Here's how the part is built. I have some questions about the finished solid (model axes, mm). A direction names the side the tool comes from. Coordinates: 2 decimals unless noted, no trailing zeros. Write each loop counter-clockwise with the first axis right and the second up, starting at its lowest first coordinate (ties: lowest second). Pieces come first, ordered by that corner, then holes.
Item 1: For faces 4 (the face through (-5.937, 13, -1)), 5 (the face through (10.444, -14.766, 1.009)), which set-ups out of +Z, -Z, +X, -X, +Y, -Y let a thin tool reach every point of the face, with its end or its side?
Item 2: If I drill on line 1 (X direction, y = -8, z = -0.5); line 2 (X direction, y = 16, z = 2.8) (3 decimals); line 3 (X direction, y = -15.5, z = 0.15), over which ranges is the centre line in solid material (lowest first)?
Item 3: If we section it at D-D (z = 3.5): Please give me the cut outline in (x, y).
Item 4: I'm going to push flat-ended pins straight in: pin 1 Ø10.5 at (x, y) = (1.5, 2.5) entering from -Z; pin 2 Ø4.5 at (x, y) = (-11.5, 1.5) entering from -Z; pin 3 Ø4.5 at (x, y) = (12.94, 14.66) entering from -Z. Where does each tip first touch, or does it pass through?
Item 5: If we section it at B-B (y = 8): Please give me the cut outline in (x, z), then the cut area to 3 significant figures.
Item 6: If we section it at A-A (x = -1.5): Please give me the cut outline in (y, z).
Item 7: We'd pull the mould along Y, two halves only. Please class faces 1 (the face through (-0.79, -11.52, 1.97)), 2 (the face through (-18.713, 0, 1)), 3 (the face through (0, -19.656, 1)): +Y half, -Y half, draft (parallel to the pull), parting line (faces both ways), or undercut.
Item 8: If we section it at C-C (z = 1.5): Please give me the cut outline in (x, y), then the cut area to 3 significant figures.
from build123d import *

# Parameters (mm, degrees)
SKETCH1_W           = 36.654989836
SKETCH1_H           = 39.3126
SKETCH1_R           = 2.15
BOSS_EXTRUDE1_DEPTH = 4
SKETCH2_W           = 36.654989836
SKETCH2_H           = 39.3126
BOSS_EXTRUDE2_DEPTH = 1.900000015
SKETCH3_R           = 2.5
CUT_EXTRUDE1_DEPTH  = 5.900000015
SKETCH4_W           = 8.8912
SKETCH4_H           = 11.10254
CUT_EXTRUDE2_DEPTH  = 3


with BuildPart() as part:
    # Sketch1 → Boss-Extrude1 (new body)
    with BuildSketch(Plane.XY):
        with Locations((-0.385705082, 0)):
            Rectangle(SKETCH1_W, SKETCH1_H)
        with Locations((-0.4826, 13.6525)):
            Circle(SKETCH1_R, mode=Mode.SUBTRACT)
        with Locations((-0.508, -13.6525)):
            Circle(SKETCH1_R, mode=Mode.SUBTRACT)
    extrude(amount=BOSS_EXTRUDE1_DEPTH)

    # Sketch2 → Boss-Extrude2 (add)
    with BuildSketch(Plane(origin=(0, 0, 0), x_dir=(-1, 0, 0), z_dir=(0, 0, -1))):
        with Locations((0.385705082, 0)):
            Rectangle(SKETCH2_W, SKETCH2_H)
        with BuildLine():
            Line((-17.1132, 10.4965), (-6.464885425, 10.4965))
            Line((-6.464885425, 10.4965), (-4.9212, 12.040185425))
            Line((-4.9212, 12.040185425), (-4.9212, 13.6525))
            ThreePointArc((-4.9212, 13.6525), (0.508, 19.0817), (5.9372, 13.6525))
            Line((5.9372, 13.6525), (5.9372, 12.040185425))
            Line((5.9372, 12.040185425), (7.480885425, 10.4965))
            Line((7.480885425, 10.4965), (17.1132, 10.4965))
            Line((17.1132, 10.4965), (17.1132, -0.0127))
            Line((17.1132, -0.0127), (17.105585288, -10.521897241))
            Line((17.105585288, -10.521897241), (7.473273242, -10.514917899))
            Line((7.473273242, -10.514917899), (5.928469705, -12.057484402))
            Line((5.928469705, -12.057484402), (5.927301461, -13.669798554))
            ThreePointArc((5.927301461, -13.669798554), (0.494169019, -19.095063262), (-4.931095689, -13.66193082))
            Line((-4.931095689, -13.66193082), (-4.929927445, -12.049616668))
            Line((-4.929927445, -12.049616668), (-6.472493947, -10.504813132))
            Line((-6.472493947, -10.504813132), (-17.120805727, -10.497097621))
            Line((-17.120805727, -10.497097621), (-17.1132, -0.000300188))
            Line((-17.1132, -0.000300188), (-17.1132, 10.4965))
        make_face(mode=Mode.SUBTRACT)
    extrude(amount=BOSS_EXTRUDE2_DEPTH)

    # Sketch3 → Cut-Extrude1 (cut)
    with BuildSketch(Plane(origin=(0, 0, -1.900000015), x_dir=(-1, 0, 0), z_dir=(0, 0, -1))):
        with Locations((-12.941789836, 14.6563)):
            Circle(SKETCH3_R)
        with Locations(Location((13.7132, 14.6563, 0), (0, 0, 180))):
            Circle(SKETCH3_R)
        with Locations((13.7132, -14.6563)):
            Circle(SKETCH3_R)
        with Locations(Location((-12.941789836, -14.6563, 0), (0, 0, 180))):
            Circle(SKETCH3_R)
    extrude(amount=-CUT_EXTRUDE1_DEPTH, mode=Mode.SUBTRACT)

    # Sketch4 → Cut-Extrude2 (cut)
    with BuildSketch(Plane(origin=(0, 0, 0), x_dir=(-1, 0, 0), z_dir=(0, 0, -1))):
        with Locations((12.2676, -0.28623)):
            Rectangle(SKETCH4_W, SKETCH4_H)
    extrude(amount=-CUT_EXTRUDE2_DEPTH, mode=Mode.SUBTRACT)


solid = part.part
Answer list:
1. face 4: -Z
1. face 5: +Z, -Z
2. line 1: x = -18.71 to -17.11, 17.12 to 17.94
2. line 2: x = -18.713 to -15.821, -11.605 to 10.834, 15.05 to 17.942
2. line 3: x = -18.71 to -16.07, -11.36 to -1.61, 0.59 to 10.59, 15.3 to 17.94
3. outline: (-18.71, -19.66) - (17.94, -19.66) - (17.94, 19.66) - (-18.71, 19.66) - close; hole circle Ø5 at (-13.71, -14.66); hole circle Ø5 at (-13.71, 14.66); hole circle Ø4.3 at (-0.51, -13.65); hole circle Ø4.3 at (-0.48, 13.65); hole circle Ø5 at (12.94, -14.66); hole circle Ø5 at (12.94, 14.66)
4. pin 1: stops at z = 0
4. pin 2: stops at z = 3
4. pin 3: passes through
5. outline: (-18.71, -1.9) - (-17.11, -1.9) - (-17.11, 0) - (17.11, 0) - (17.11, -1.9) - (17.94, -1.9) - (17.94, 4) - (-18.71, 4) - close
5. area: 151 mm2
6. outline: (-19.66, -1.9) - (-19, -1.9) - (-19, 0) - (-15.56, 0) - (-15.56, 4) - (-19.66, 4) - close; (-11.75, 0) - (11.76, 0) - (11.76, 4) - (-11.75, 4) - close; (15.55, 0) - (18.99, 0) - (18.99, -1.9) - (19.66, -1.9) - (19.66, 4) - (15.55, 4) - close
7. face 1: undercut
7. face 2: draft
7. face 3: -Y half
8. outline: (-18.71, -19.66) - (17.94, -19.66) - (17.94, 19.66) - (-18.71, 19.66) - close; hole (-16.71, -5.84) - (-7.82, -5.84) - (-7.82, 5.27) - (-16.71, 5.27) - close; hole circle Ø5 at (-13.71, -14.66); hole circle Ø5 at (-13.71, 14.66); hole circle Ø4.3 at (-0.51, -13.65); hole circle Ø4.3 at (-0.48, 13.65); hole circle Ø5 at (12.94, -14.66); hole circle Ø5 at (12.94, 14.66)
8. area: 1,230 mm2
